from build123d import *

# Parameters (mm, degrees)
SKETCH_1_R      = 2
EXTRUDE_1_DEPTH = 10
EXTRUDE_START   = 7
EXTRUDE_3_DEPTH = 3


with BuildPart() as part:
    # Эскиз1 → Бобышка-Вытянуть1 (new body)
    with BuildSketch(Plane(origin=(0, 0, 0), x_dir=(1, 0, 0), z_dir=(0, 1, 0))):
        with BuildLine():
            Line((-26, 29), (26, 29))
            ThreePointArc((26, 29), (30.242640687, 27.242640687), (32, 23))
            Line((32, 23), (32, -23))
            ThreePointArc((32, -23), (30.242640687, -27.242640687), (26, -29))
            Line((26, -29), (-26, -29))
            ThreePointArc((-26, -29), (-30.242640687, -27.242640687), (-32, -23))
            Line((-32, -23), (-32, 23))
            ThreePointArc((-32, 23), (-30.242640687, 27.242640687), (-26, 29))
        make_face()
        with Locations(Location((-26, 23, 0), (0, 0, 270))):
            Circle(SKETCH_1_R, mode=Mode.SUBTRACT)
        with Locations(Location((26, 23, 0), (0, 0, 90))):
            Circle(SKETCH_1_R, mode=Mode.SUBTRACT)
        with Locations(Location((26, -23, 0), (0, 0, 270))):
            Circle(SKETCH_1_R, mode=Mode.SUBTRACT)
        with Locations(Location((-26, -23, 0), (0, 0, 90))):
            Circle(SKETCH_1_R, mode=Mode.SUBTRACT)
        with BuildLine():
            Line((7.75, 26), (-16.75, 26))
            ThreePointArc((-16.75, 26), (-18.871320344, 25.121320344), (-19.75, 23))
            ThreePointArc((-19.75, 23), (-21.580582618, 18.580582618), (-26, 16.75))
            ThreePointArc((-26, 16.75), (-28.121320344, 15.871320344), (-29, 13.75))
            Line((-29, 13.75), (-29, -13.75))
            ThreePointArc((-29, -13.75), (-28.121320344, -15.871320344), (-26, -16.75))
            Line((-26, -16.75), (-17, -16.75))
            ThreePointArc((-17, -16.75), (-12.580582618, -18.580582618), (-10.75, -23))
            ThreePointArc((-10.75, -23), (-9.871320344, -25.121320344), (-7.75, -26))
            Line((-7.75, -26), (16.75, -26))
            ThreePointArc((16.75, -26), (18.871320344, -25.121320344), (19.75, -23))
            ThreePointArc((19.75, -23), (21.580582618, -18.580582618), (26, -16.75))
            ThreePointArc((26, -16.75), (28.121320344, -15.871320344), (29, -13.75))
            Line((29, -13.75), (29, 13.75))
            ThreePointArc((29, 13.75), (28.121320344, 15.871320344), (26, 16.75))
            Line((26, 16.75), (17, 16.75))
            ThreePointArc((17, 16.75), (12.580582618, 18.580582618), (10.75, 23))
            ThreePointArc((10.75, 23), (9.871320344, 25.121320344), (7.75, 26))
        make_face(mode=Mode.SUBTRACT)
        with BuildLine():
            Line((17, 18.75), (23.366086562, 18.75))
            ThreePointArc((23.366086562, 18.75), (21.020896599, 22.543349889), (22.636965656, 26.7))
            Line((22.636965656, 26.7), (11.113034344, 26.7))
            ThreePointArc((11.113034344, 26.7), (12.322481368, 25.022971611), (12.75, 23))
            ThreePointArc((12.75, 23), (13.99479618, 19.99479618), (17, 18.75))
        make_face(mode=Mode.SUBTRACT)
        with BuildLine():
            Line((-22.636965656, -26.7), (-11.113034344, -26.7))
            ThreePointArc((-11.113034344, -26.7), (-12.322481368, -25.022971611), (-12.75, -23))
            ThreePointArc((-12.75, -23), (-13.99479618, -19.99479618), (-17, -18.75))
            Line((-17, -18.75), (-23.366086562, -18.75))
            ThreePointArc((-23.366086562, -18.75), (-21.020896599, -22.543349889), (-22.636965656, -26.7))
        make_face(mode=Mode.SUBTRACT)
    extrude(amount=EXTRUDE_1_DEPTH)

    # Эскиз1<15> → Бобышка-Вытянуть3 (add)
    with BuildSketch(Plane(origin=(0, 0, 0), x_dir=(1, 0, 0), z_dir=(0, 1, 0)).offset(EXTRUDE_START)):
        with BuildLine():
            ThreePointArc((-17, -16.75), (-12.580582618, -18.580582618), (-10.75, -23))
            ThreePointArc((-10.75, -23), (-9.871320344, -25.121320344), (-7.75, -26))
            Line((-7.75, -26), (16.75, -26))
            ThreePointArc((16.75, -26), (18.871320344, -25.121320344), (19.75, -23))
            ThreePointArc((19.75, -23), (21.580582618, -18.580582618), (26, -16.75))
            ThreePointArc((26, -16.75), (28.121320344, -15.871320344), (29, -13.75))
            Line((29, -13.75), (29, 13.75))
            ThreePointArc((29, 13.75), (28.121320344, 15.871320344), (26, 16.75))
            Line((26, 16.75), (17, 16.75))
            ThreePointArc((17, 16.75), (12.580582618, 18.580582618), (10.75, 23))
            ThreePointArc((10.75, 23), (9.871320344, 25.121320344), (7.75, 26))
            Line((7.75, 26), (-16.75, 26))
            ThreePointArc((-16.75, 26), (-18.871320344, 25.121320344), (-19.75, 23))
            ThreePointArc((-19.75, 23), (-21.580582618, 18.580582618), (-26, 16.75))
            ThreePointArc((-26, 16.75), (-28.121320344, 15.871320344), (-29, 13.75))
            Line((-29, 13.75), (-29, -13.75))
            ThreePointArc((-29, -13.75), (-28.121320344, -15.871320344), (-26, -16.75))
            Line((-26, -16.75), (-17, -16.75))
        make_face()
        with BuildLine():
            ThreePointArc((12.75, 23), (12.322481368, 25.022971611), (11.113034344, 26.7))
            Line((11.113034344, 26.7), (22.636965656, 26.7))
            ThreePointArc((22.636965656, 26.7), (21.020896599, 22.543349889), (23.366086562, 18.75))
            Line((23.366086562, 18.75), (17, 18.75))
            ThreePointArc((17, 18.75), (13.99479618, 19.99479618), (12.75, 23))
        make_face()
        with BuildLine():
            ThreePointArc((-12.75, -23), (-12.322481368, -25.022971611), (-11.113034344, -26.7))
            Line((-11.113034344, -26.7), (-22.636965656, -26.7))
            ThreePointArc((-22.636965656, -26.7), (-21.020896599, -22.543349889), (-23.366086562, -18.75))
            Line((-23.366086562, -18.75), (-17, -18.75))
            ThreePointArc((-17, -18.75), (-13.99479618, -19.99479618), (-12.75, -23))
        make_face()
    extrude(amount=EXTRUDE_3_DEPTH)


solid = part.part
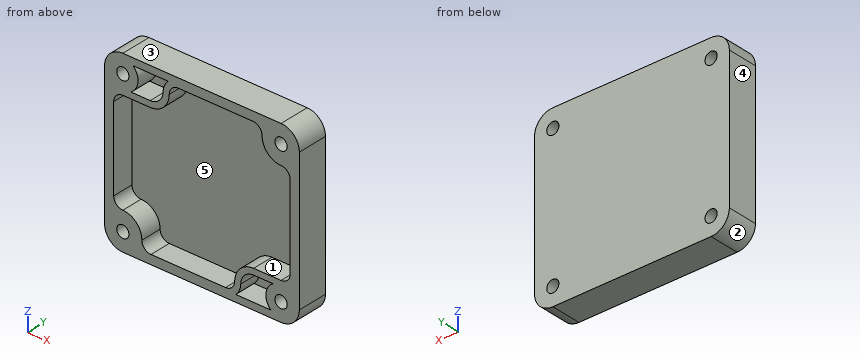
Check sheet for the modelled part. Datum: model origin and axes. Units: mm. Face numbers are marked on the shaded views. A direction names the side the tool comes from. Coordinates: 2 decimals unless noted, no trailing zeros. Write each loop counter-clockwise with the first axis right and the second up, starting at its lowest first coordinate (ties: lowest second). Pieces come first, ordered by that corner, then holes.
Item 1: Cross-section at D-D on z = 24. Record the boundary of the cut face in (x, y), then the cut area to 3 significant figures.
Numbers:
outline: (-31.92, 0) - (-27.73, 0) - (-27.73, 10) - (-31.92, 10) - close; (-24.27, 0) - (-21.1, 0) - (-21.1, 7) - (-12.65, 7) - (-12.65, 0) - (-10.58, 0) - (-10.58, 7) - (19.58, 7) - (19.58, 0) - (24.27, 0) - (24.27, 10) - (-24.27, 10) - close; (27.73, 0) - (31.92, 0) - (31.92, 10) - (27.73, 10) - close
area: 299 mm2
Item 2: Cross-section at C-C on z = -3. Record the boundary of the cut face in (x, y).
Numbers:
outline: (-32, 0) - (-29, 0) - (-29, 7) - (29, 7) - (29, 0) - (32, 0) - (32, 10) - (-32, 10) - close
Item 3: Cross-section at B-B on x = 2.5. Record the boundary of the cut face in (y, z).
Numbers:
outline: (0, -29) - (10, -29) - (10, 29) - (0, 29) - (0, 26) - (7, 26) - (7, -26) - (0, -26) - close
Item 4: Access from +Z, -Z, +X, -X, +Y, -Y to the whole of each face (thin tool, end or side, straight path). Record for the marked faces 4 and 5.
Numbers:
face 4: +Z, -Z, -X, +Y, -Y
face 5: -Y
Item 5: Cross-section at A-A on y = 8.5. Record the boundary of the cut face in (x, z), then the cut area to 3 significant figures.
Numbers:
outline: (-32, -23) arc R6 ccw to (-26, -29) - (26, -29) arc R6 ccw to (32, -23) - (32, 23) arc R6 ccw to (26, 29) - (-26, 29) arc R6 ccw to (-32, 23) - close; hole circle Ø4 at (-26, -23); hole circle Ø4 at (-26, 23); hole circle Ø4 at (26, -23); hole circle Ø4 at (26, 23)
area: 3,630 mm2
Item 6: Scan lines: probe 1 along X at (y, z) = (3, -23); probe 2 along Z at (x, y) = (-19, 2); probe 3 along X at (y, z) = (5.75, 23). Record each from-to range of solid material in increasing order.
Numbers:
probe 1: x = -32 to -28, -24 to -19.75, 10.75 to 12.75, 21 to 24, 28 to 32
probe 2: z = -29 to -24.98, 16.75 to 18.75, 26.7 to 29
probe 3: x = -32 to -28, -24 to -21, -12.75 to -10.75, 19.75 to 24, 28 to 32
Item 7: Mould release check, pull along X, two halves, no side actions. Record for the marked faces 1, 2 and 3: released by +X, released by -X, zero draft, split by the parting line, or undercut.
Numbers:
face 1: undercut
face 2: released by -X
face 3: zero draft
Item 8: Depth check by flat-ended pin: pin 1 Ø4 at (x, z) = (-0.5, -14.5) entering from -Y; pin 2 Ø3 at (x, z) = (-26, 23) entering from +Y. Enter the tip coordinate at first touch or a pass-through.
Numbers:
pin 1: stops at y = 7
pin 2: passes through
